Geometry: final body of the model. Coordinates: model frame, mm. Face numbers are marked on the shaded views. Coordinates: 2 decimals unless noted, no trailing zeros. Loops run counter-clockwise (first coordinate to the right, second up) from the corner with the lowest first, then second, coordinate; pieces in that order, holes last. Notation, with made-up numbers: M 68.5,39 L 120.5,39 A13 cw 120.5,52 Z; hole C 79.5,-32 d4. An arc over 180 degrees is marked long. Write each question's results on one line, items separated by ' | '. Start each with the question number.
from build123d import *

# Parameters (mm, degrees)
MAIN_BODY_DEPTH           = 120
LOCKING_MECHANISM_DEPTH   = 120
LOCKING_MECHANISM_2_DEPTH = 120


with BuildPart() as part:
    # Curve → Main Body (new body)
    with BuildSketch(Plane.XY):
        with BuildLine():
            ThreePointArc((-85, 0), (-47.139087644, -70.731226598), (32.715445084, -78.451893877))
            Line((32.715445084, -78.451893877), (34.63988303, -83.066711164))
            ThreePointArc((34.63988303, -83.066711164), (-49.911975153, -74.891886986), (-90, 0))
            Line((-90, 0), (-85, 0))
        make_face()
    extrude(amount=MAIN_BODY_DEPTH)

    # Lock shape → Locking Mechanism (add)
    with BuildSketch(Plane.XY.offset(120)):
        with BuildLine():
            Line((32.715445084, -78.451893877), (39.955604844, -73.060549627))
            ThreePointArc((39.955604844, -73.060549627), (40.81748466, -72.898257413), (41.475815628, -73.477719162))
            Line((41.475815628, -73.477719162), (44.338781633, -80.343134095))
            ThreePointArc((44.338781633, -80.343134095), (44.287191647, -81.218641979), (43.565362465, -81.716776713))
            Line((43.565362465, -81.716776713), (34.63988303, -83.066711164))
            Line((34.63988303, -83.066711164), (32.715445084, -78.451893877))
        make_face()
    extrude(amount=-LOCKING_MECHANISM_DEPTH)

    # Lock shape 2 → Locking Mechanism 2 (add)
    with BuildSketch(Plane.XY.offset(120)):
        with BuildLine():
            Line((-90, 0), (-92.189366094, 8.757464375))
            ThreePointArc((-92.189366094, 8.757464375), (-92.007429032, 9.615412209), (-91.219223594, 10))
            Line((-91.219223594, 10), (-83.780776406, 10))
            ThreePointArc((-83.780776406, 10), (-82.992570968, 9.615412209), (-82.810633906, 8.757464375))
            Line((-82.810633906, 8.757464375), (-85, 0))
            Line((-85, 0), (-90, 0))
        make_face()
    extrude(amount=-LOCKING_MECHANISM_2_DEPTH)


solid = part.part
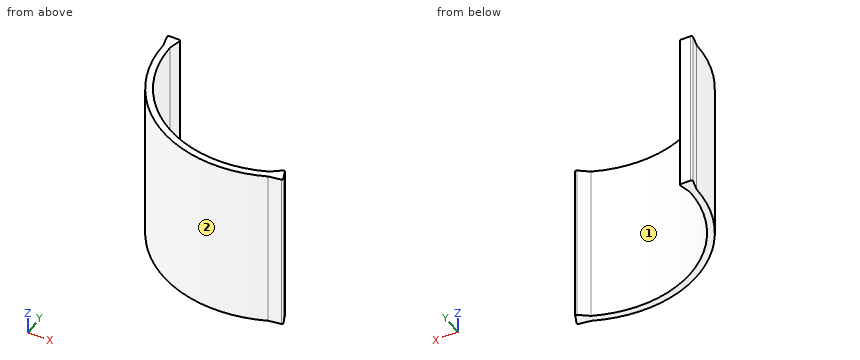
Item 1: Section C-C, the plane x = -12. Return loops of the section in (y, z), plus the area to 3 significant figures.
Item 2: Section B-B, the plane y = 3. Return loops of the section in (x, z), plus the area to 3 significant figures.
Item 3: Contact query for flat-ended pins moving along their axis: P1, Ø1.5, axis at y = -58, z = 65.5, coming from the +X side; P2, Ø8, axis at x = -54, z = 58.5, coming from the -Y side; P3, Ø6, axis at x = 30.5, z = 19.5, coming from the -Y side. Output: stop coordinate, or through.
Item 4: Section A-A, the plane z = 63.5. Return loops of the section in (x, y), plus the area to 3 significant figures.
Item 5: Ray query, L1, parallel to Y at x = -52, z = 85.5; L2, parallel to X at y = 4, z = 70; L3, parallel to X at y = -24, z = 99.5. Return the intervals inside material, ascending. Write a range as [from, to].
Item 6: Pull-direction query (X, two-part tool) for the marked faces 1 and 2; classes: released by +X, released by -X, zero draft, split by the parting line, or undercut.
Solutions:
1) outline: M -89.2,0 L -84.15,0 L -84.15,120 L -89.2,120 Z | area: 606 mm²
2) outline: M -90.75,0 L -84.25,0 L -84.25,120 L -90.75,120 Z | area: 780 mm²
3) P1: stops at x = -61.43 | P2: stops at y = -74.83 | P3: stops at y = -85.7
4) outline: M -92.19,8.76 L -90,0 A90 ccw 34.64,-83.07 L 43.57,-81.72 A1 ccw 44.34,-80.34 L 41.48,-73.48 A1 ccw 39.96,-73.06 L 32.72,-78.45 A85 cw -85,0 L -82.81,8.76 A1 ccw -83.78,10 L -91.22,10 A1 ccw Z | area: 1,010 mm²
5) L1: y = [-73.46, -67.24] | L2: x = [-91, -84] | L3: x = [-86.74, -81.54]
6) face 1: undercut | face 2: split by the parting line
